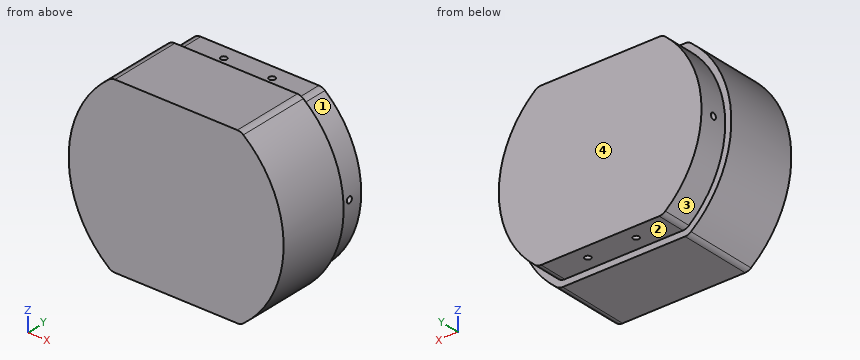
from build123d import *

# Parameters (mm, degrees)
Y_KSEKLIK_EKSTR_ZYON1_DEPTH = 53
KES_EKSTR_ZYON1_START       = -15
KES_EKSTR_ZYON1_DEPTH       = 15
M3_BO_LUKLU_DELIK2_D        = 3.2
M3_BO_LUKLU_DELIK2_DEPTH    = 6.9
M3_BO_LUKLU_DELIK2_TIP      = 0.96137699
M3_BO_LUKLU_DELIK1_D        = 3.2
M3_BO_LUKLU_DELIK1_DEPTH    = 6.9
M3_BO_LUKLU_DELIK1_TIP      = 0.96137699
RADYUS1_R                   = 5
DAIRESEL_KAPLAMA1_COUNT     = 2
DAIRESEL_KAPLAMA1_ANGLE     = 180


with BuildPart() as part:
    # Çizim1 → Yükseklik-Ekstrüzyon1 (new body)
    with BuildSketch(Plane(origin=(0, 0, 0), x_dir=(1, 0, 0), z_dir=(0, 1, 0))):
        with BuildLine():
            Line((-32.040014045, 45), (32.040014045, 45))
            ThreePointArc((32.040014045, 45), (33.696486936, 44.717636862), (35.165869074, 43.902439024))
            ThreePointArc((35.165869074, 43.902439024), (56.25, 0), (35.165869074, -43.902439024))
            ThreePointArc((35.165869074, -43.902439024), (33.696486936, -44.717636862), (32.040014045, -45))
            Line((32.040014045, -45), (-32.040014045, -45))
            ThreePointArc((-32.040014045, -45), (-33.696486936, -44.717636862), (-35.165869074, -43.902439024))
            ThreePointArc((-35.165869074, -43.902439024), (-56.25, 0), (-35.165869074, 43.902439024))
            ThreePointArc((-35.165869074, 43.902439024), (-33.696486936, 44.717636862), (-32.040014045, 45))
        make_face()
    extrude(amount=Y_KSEKLIK_EKSTR_ZYON1_DEPTH)

    # Çizim2 → Kes-Ekstrüzyon1 (cut)
    with BuildSketch(Plane(origin=(0, 53, 0), x_dir=(1, 0, 0), z_dir=(0, 1, 0)).offset(KES_EKSTR_ZYON1_START)):
        with BuildLine():
            Line((33.75, 45), (-33.75, 45))
            ThreePointArc((-33.75, 45), (-56.25, 0), (-33.75, -45))
            Line((-33.75, -45), (33.75, -45))
            ThreePointArc((33.75, -45), (56.25, 0), (33.75, 45))
        make_face()
        with BuildLine():
            Line((32.665922611, -41.8), (-32.665922611, -41.8))
            ThreePointArc((-32.665922611, -41.8), (-53.05, 0), (-32.665922611, 41.8))
            Line((-32.665922611, 41.8), (32.665922611, 41.8))
            ThreePointArc((32.665922611, 41.8), (53.05, 0), (32.665922611, -41.8))
        make_face(mode=Mode.SUBTRACT)
    extrude(amount=KES_EKSTR_ZYON1_DEPTH, mode=Mode.SUBTRACT)

    # M3 Boşluklu Delik2
    with Locations(Plane(origin=(0, 0, -41.8), x_dir=(-1, 0, 0), z_dir=(0, 0, -1))):
        with Locations((12.665922611, 45.5), (-12.665922611, 45.5)):
            Hole(M3_BO_LUKLU_DELIK2_D / 2, depth=M3_BO_LUKLU_DELIK2_DEPTH)
            with Locations((0, 0, -(M3_BO_LUKLU_DELIK2_DEPTH + M3_BO_LUKLU_DELIK2_TIP / 2))):  # 118° drill point
                Cone(0, M3_BO_LUKLU_DELIK2_D / 2, M3_BO_LUKLU_DELIK2_TIP, mode=Mode.SUBTRACT)

    # M3 Boşluklu Delik1
    with Locations(Plane.XY.offset(41.8)):
        with Locations((12.665922611, 45.5), (-12.665922611, 45.5)):
            Hole(M3_BO_LUKLU_DELIK1_D / 2, depth=M3_BO_LUKLU_DELIK1_DEPTH)
            with Locations((0, 0, -(M3_BO_LUKLU_DELIK1_DEPTH + M3_BO_LUKLU_DELIK1_TIP / 2))):  # 118° drill point
                Cone(0, M3_BO_LUKLU_DELIK1_D / 2, M3_BO_LUKLU_DELIK1_TIP, mode=Mode.SUBTRACT)

    # Radyus1
    radyus1_edges = [part.edges().sort_by_distance(p)[0] for p in [
        (-32.665922611, 45.5, -41.8),
        (32.665922611, 45.5, -41.8),
        (32.665922611, 45.5, 41.8),
        (-32.665922611, 45.5, 41.8),
    ]]
    fillet(radyus1_edges, radius=RADYUS1_R)

    # Çizim19 → M3 Boşluklu Delik3 (revolve, cut)
    with BuildSketch(Plane(origin=(53.05, 45.5, 0), x_dir=(0, 0, -1), z_dir=(0, 1, 0))):
        Polygon((0, 0), (0, 12.76137699), (1.6, 11.8), (1.6, 0), align=None)
    m3_bo_luklu_delik3 = revolve(axis=Axis((59.4, 45.5, 0), (-1, 0, 0)), mode=Mode.SUBTRACT)

    # Dairesel Kaplama1: M3 Boşluklu Delik3 ×2 about axis
    dairesel_kaplama1_axis = Axis((0, 53, 0), (0, 1, 0))
    for i in range(1, DAIRESEL_KAPLAMA1_COUNT):
        add(m3_bo_luklu_delik3.rotate(dairesel_kaplama1_axis, i * DAIRESEL_KAPLAMA1_ANGLE / (DAIRESEL_KAPLAMA1_COUNT - 1)), mode=Mode.SUBTRACT)


solid = part.part
Part model, mm, in its own coordinate system. Face numbers are marked on the shaded views. A direction names the side the tool comes from. Coordinates: 2 decimals unless noted, no trailing zeros. Write each loop counter-clockwise with the first axis right and the second up, starting at its lowest first coordinate (ties: lowest second). Pieces come first, ordered by that corner, then holes. Notation, with made-up numbers: M -16,16.25 L 30,16.25 A17 ccw 30,27.25 Z; hole C 65.25,53 d4. An arc over 180 degrees is marked long. Return JSON: item names as keys, results as strings.
1. 3-axis set-ups, long thin cutter, end or side, ignore diameter. For the marked faces 1, 2, 3 and 4: which of +Z, -Z, +X, -X, +Y, -Y reach the whole face in a straight line?
Determined:
{"face 1": "+X, +Y", "face 2": "-Z, +X, -X, +Y", "face 3": "-X, +Y", "face 4": "+Z, -Z, +X, -X, +Y"}
2. Probe L1, parallel to Y at x = -47.5, z = 0; L2, parallel to X at y = 45.5, z = 36.5; L3, parallel to X at y = 45.5, z = 38.5. List the from-to ranges inside material, lowest first.
Determined:
{"L1": "0 to 43.9, 47.1 to 53", "L2": "-38.5 to -14.27, -11.07 to 11.07, 14.27 to 38.5", "L3": "-36.5 to -14.27, -11.07 to 11.07, 14.27 to 36.5"}
3. Saw through at B-B, the plane z = -36.5. Write the cut outline in (x, y), then the cut area to 3 significant figures.
Determined:
{"outline": "M -42.8,0 L 42.8,0 L 42.8,38 L 38.5,38 L 38.5,53 L -38.5,53 L -38.5,38 L -42.8,38 Z; hole C -12.67,45.5 d3.2; hole C 12.67,45.5 d3.2", "area": "4,390 mm²"}
4. Flat gauge pins, fed straight in: pin 1 Ø6 at (x, y) = (-44.5, 36.5) entering from -Z; pin 2 Ø4 at (x, y) = (-44, 42) entering from +Z; pin 3 Ø5 at (y, z) = (11.5, -16) entering from +X. Where does each tip first touch, or does it go through?
Determined:
{"pin 1": "z = -37.97", "pin 2": "z = 32.41", "pin 3": "x = 54.61"}
5. Saw through at C-C, the plane x = 16. Write the cut outline in (y, z).
Determined:
{"outline": "M 0,-45 L 38,-45 L 38,-41.8 L 53,-41.8 L 53,41.8 L 38,41.8 L 38,45 L 0,45 Z"}
6. Saw through at A-A, the plane y = 49. Write the cut outline in (x, z), then the cut area to 3 significant figures.
Determined:
{"outline": "M -34.11,-40.63 A5 ccw -30.9,-41.8 L 30.9,-41.8 A5 ccw 34.11,-40.63 A53.05 ccw 34.11,40.63 A5 ccw 30.9,41.8 L -30.9,41.8 A5 ccw -34.11,40.63 A53.05 ccw Z", "area": "7,840 mm²"}
